Part model, mm, in its own coordinate system. A direction names the side the tool comes from. Round coordinates to 2 decimals unless told otherwise and drop trailing zeros. Write each loop counter-clockwise with the first axis right and the second up, starting at its lowest first coordinate (ties: lowest second). Pieces come first, ordered by that corner, then holes. Notation, with made-up numbers: (69.25, 84.25) -> (128.25, 84.25) arc R29 ccw to (128.25, 117.25) -> close; hole circle Ø8 at (59, 1). An arc over 180 degrees is marked (long way). Return JSON: item names as keys, results as strings. Group by question number.
(1) Saw through at A-A (z = 0.65). List the corners of the cut face in (x, y), plus the area to 3 significant figures.
(2) Tool access for faces 4 (the flat face through (0, 1, -2)), 5 (the flat face through (0.68, 56.52, 2.73)): list every direction of +Z, -Z, +X, -X, +Y, -Y with a clear straight run to the whole face (end or side of a thin tool).
(3) Saw through at B-B (y = -31). List the corners of the cut face in (x, z).
(4) Mould opens along Y. For faces 1 (the flat face through (0.68, -56.52, 2.73)), 2 (the cylindrical face through (0, 58, 3)), 3 (the flat face through (0, -58.42, 0)) say: +Y half, -Y half, draft (parallel to the pull), parting line (faces both ways), or undercut.
(5) Drop a flat-ended pin along its axis: pin 1 Ø1.5 at (y, z) = (15, 1) entering from -X. Give the stop position or say it passes through.
(6) Drill centre lines: L1, parallel to Z at x = 2, y = -15; L2, parallel to X at y = -48.5, z = -0.25; L3, parallel to Z at x = -2.7, y = 34. Where is each one in solid material? Low to high. Write a range as from..to.
from build123d import *

# Parameters (mm, degrees)
BOSS_EXTRUDE1_DEPTH = 58.42
SKETCH2_W           = 0.35
SKETCH2_H           = 0.9


with BuildPart() as part:
    # Sketch1 → Boss-Extrude1 (new body, symmetric)
    with BuildSketch(Plane(origin=(0, 0, 0), x_dir=(1, 0, 0), z_dir=(0, 1, 0))):
        with BuildLine():
            Line((-2.236067977, 2), (2.236067977, 2))
            ThreePointArc((2.236067977, 2), (0, -3), (-2.236067977, 2))
        make_face()
    extrude(amount=BOSS_EXTRUDE1_DEPTH, both=True)

    # Sketch2 → Cut-Revolve1 (revolve, cut)
    with BuildSketch(Plane.XY):
        with Locations((2.825, 56.97)):
            Rectangle(SKETCH2_W, SKETCH2_H)
        with Locations((2.825, -56.97)):
            Rectangle(SKETCH2_W, SKETCH2_H)
    revolve(axis=Axis((0, 48.05613995, 0), (0, -1, 0)), mode=Mode.SUBTRACT)


solid = part.part
Computed values:
{
 "1": {"outline": "(-2.93, -58.42) -> (2.93, -58.42) -> (2.93, -57.42) -> (2.57, -57.42) -> (2.57, -56.52) -> (2.93, -56.52) -> (2.93, 56.52) -> (2.57, 56.52) -> (2.57, 57.42) -> (2.93, 57.42) -> (2.93, 58.42) -> (-2.93, 58.42) -> (-2.93, 57.42) -> (-2.57, 57.42) -> (-2.57, 56.52) -> (-2.93, 56.52) -> (-2.93, -56.52) -> (-2.57, -56.52) -> (-2.57, -57.42) -> (-2.93, -57.42) -> close", "area": "683 mm2"},
 "2": {"face 4": "-Z, +X, -X, +Y, -Y", "face 5": "none"},
 "3": {"outline": "(-2.24, -2) -> (2.24, -2) arc R3 ccw (long way) to start"},
 "4": {"face 1": "undercut", "face 2": "draft", "face 3": "-Y half"},
 "5": {"pin 1": "x = -2.99"},
 "6": {"L1": "-2..2.24", "L2": "-2.99..2.99", "L3": "-1.31..1.31"}
}
